Verification items for the finished model (mm, model axes). A direction names the side the tool comes from. Coordinates: 2 decimals unless noted, no trailing zeros. Loops run counter-clockwise (first coordinate to the right, second up) from the corner with the lowest first, then second, coordinate; pieces in that order, holes last. Notation, with made-up numbers: (11.25, 59.25) - (18.25, 59.25) arc R7 cw to (18.25, 71.25) - close; hole circle Ø10 at (33, -0.5). An arc over 180 degrees is marked (long way). One line per item, written item: value. Start each with the question number.
(1) Thickness scan on probe 1 along X at (y, z) = (-2.75, 6.5); probe 2 along Y at (x, z) = (-2.5, 17.5). Record the ranges inside material, lowest first. Write a range as [from, to].
(2) Section check B-B (x = -9). Record the boundary of the cut face in (y, z), plus the area to 3 significant figures.
(3) Section check C-C (z = 10.5). Record the boundary of the cut face in (x, y).
(4) Draft check along Y on faces 3 (the face through (-32.75, 0, 10)), 4 (the face through (0, 6.1, 10)), 5 (the face through (0, 3.1, 10)). Enter one of: +Y half, -Y half, draft (parallel to the pull), parting line (faces both ways), or undercut.
(5) Set-up check for faces 1 (the face through (32.75, 0, 10)), 2 (the face through (-25.75, 0, 10)): record each of +Z, -Z, +X, -X, +Y, -Y from which the full face is reachable in a straight line by a thin tool's end or side.
(6) Section check A-A (y = 1.5). Record the boundary of the cut face in (x, z), plus the area to 3 significant figures.
```python
from build123d import *

# Parameters (mm, degrees)
SKETCH_W     = 65.5
SKETCH_H     = 12.2
PAD_DEPTH    = 20
SKETCH001_W  = 51.5
SKETCH001_H  = 6.2
POCKET_DEPTH = 20
CHAMFER_SIZE = 1


with BuildPart() as part:
    # Sketch → Pad (new body)
    with BuildSketch(Plane.XY):
        Rectangle(SKETCH_W, SKETCH_H)
    extrude(amount=PAD_DEPTH)

    # Sketch001 (on Face6 of Pad) → Pocket (cut)
    with BuildSketch(Plane.XY.offset(20)):
        Rectangle(SKETCH001_W, SKETCH001_H)
    extrude(amount=-POCKET_DEPTH, mode=Mode.SUBTRACT)

    # Chamfer
    chamfer_edges = [part.edges().sort_by_distance(p)[0] for p in [
        (32.75, -6.1, 10),
        (-32.75, -6.1, 10),
        (0, -6.1, 0),
        (0, -6.1, 20),
        (-32.75, 6.1, 10),
        (32.75, 6.1, 10),
        (0, 6.1, 0),
        (0, 6.1, 20),
        (32.75, 0, 20),
        (32.75, 0, 0),
        (-32.75, 0, 0),
        (-32.75, 0, 20),
        (-25.75, 0, 20),
        (0, -3.1, 20),
        (25.75, 0, 20),
        (0, 3.1, 20),
        (-25.75, 0, 0),
        (0, -3.1, 0),
        (25.75, 0, 0),
        (0, 3.1, 0),
    ]]
    chamfer(chamfer_edges, length=CHAMFER_SIZE)


solid = part.part
```
Responses:
1. probe 1: x = [-32.75, -25.75], [25.75, 32.75]
1. probe 2: y = [-6.1, -3.1], [3.1, 6.1]
2. outline: (-6.1, 1) - (-5.1, 0) - (-4.1, 0) - (-3.1, 1) - (-3.1, 19) - (-4.1, 20) - (-5.1, 20) - (-6.1, 19) - close; (3.1, 1) - (4.1, 0) - (5.1, 0) - (6.1, 1) - (6.1, 19) - (5.1, 20) - (4.1, 20) - (3.1, 19) - close
2. area: 116 mm²
3. outline: (-32.75, -5.1) - (-31.75, -6.1) - (31.75, -6.1) - (32.75, -5.1) - (32.75, 5.1) - (31.75, 6.1) - (-31.75, 6.1) - (-32.75, 5.1) - close; hole (-25.75, -3.1) - (25.75, -3.1) - (25.75, 3.1) - (-25.75, 3.1) - close
4. face 3: draft
4. face 4: +Y half
4. face 5: undercut
5. face 1: +Z, -Z, +X, +Y, -Y
5. face 2: +Z, -Z
6. outline: (-32.75, 1) - (-31.75, 0) - (-26.75, 0) - (-25.75, 1) - (-25.75, 19) - (-26.75, 20) - (-31.75, 20) - (-32.75, 19) - close; (25.75, 1) - (26.75, 0) - (31.75, 0) - (32.75, 1) - (32.75, 19) - (31.75, 20) - (26.75, 20) - (25.75, 19) - close
6. area: 276 mm²
